Design review of the part built by this model. Coordinates are the model's own, in mm. Give positions to 0.01 mm unless a question says otherwise; leave off trailing zeros. Write each loop counter-clockwise with the first axis right and the second up, starting at its lowest first coordinate (ties: lowest second). Pieces come first, ordered by that corner, then holes. Notation, with made-up numbers: M -15,-13.5 L 5,-13.5 A14 ccw 5,-0.5 Z; hole C -9,-2 d6. An arc over 180 degrees is marked long. Answer in a Markdown table with one row per item.
```python
from build123d import *

# Parameters (mm, degrees)
BOARD_OUTLINE_DEPTH = 0.508
SKETCH2_R           = 0.0762
NPTH_DEPTH          = 1.508
SKETCH3_R           = 0.405
SKETCH3_R_2         = 1.27
PTH_DEPTH           = 1.508


with BuildPart() as part:
    # Sketch1 → Board_Outline (new body)
    with BuildSketch(Plane.XY):
        Polygon((0, 0), (0, 21.59), (0.3175, 23.1775), (14.2875, 23.1775), (14.605, 21.59), (14.605, 0), align=None)
    extrude(amount=BOARD_OUTLINE_DEPTH)

    # Sketch2 → NPTH (cut, through all)
    with BuildSketch(Plane.XY):
        with Locations((1.4224, 20.3073)):
            Circle(SKETCH2_R)
        with Locations((8.5344, 4.5593)):
            Circle(SKETCH2_R)
        with Locations((12.7, 17.5641)):
            Circle(SKETCH2_R)
        with Locations((12.065, 8.4582)):
            Circle(SKETCH2_R)
        with Locations((13.2842, 7.3406)):
            Circle(SKETCH2_R)
        with Locations((0.635, 14.732)):
            Circle(SKETCH2_R)
        with Locations((3.1496, 20.4089)):
            Circle(SKETCH2_R)
        with Locations((2.4384, 14.9225)):
            Circle(SKETCH2_R)
        with Locations((2.54, 20.4089)):
            Circle(SKETCH2_R)
        with Locations((2.54, 17.3609)):
            Circle(SKETCH2_R)
        with Locations((3.7592, 20.4089)):
            Circle(SKETCH2_R)
        with Locations((2.032, 14.4145)):
            Circle(SKETCH2_R)
        with Locations((4.3688, 20.4089)):
            Circle(SKETCH2_R)
        with Locations((2.4384, 13.9065)):
            Circle(SKETCH2_R)
        with Locations((5.08, 20.4089)):
            Circle(SKETCH2_R)
        with Locations((2.4384, 13.2969)):
            Circle(SKETCH2_R)
        with Locations((5.6896, 20.4089)):
            Circle(SKETCH2_R)
        with Locations((2.4384, 12.6873)):
            Circle(SKETCH2_R)
        with Locations((6.2992, 20.4089)):
            Circle(SKETCH2_R)
        with Locations((2.032, 12.1793)):
            Circle(SKETCH2_R)
        with Locations((6.9088, 20.4089)):
            Circle(SKETCH2_R)
        with Locations((2.4384, 11.6713)):
            Circle(SKETCH2_R)
        with Locations((7.62, 20.4089)):
            Circle(SKETCH2_R)
        with Locations((12.192, 11.6713)):
            Circle(SKETCH2_R)
        with Locations((12.0904, 20.4089)):
            Circle(SKETCH2_R)
        with Locations((12.0904, 17.4625)):
            Circle(SKETCH2_R)
        with Locations((11.4808, 20.4089)):
            Circle(SKETCH2_R)
        with Locations((12.192, 14.9225)):
            Circle(SKETCH2_R)
        with Locations((10.8712, 20.4089)):
            Circle(SKETCH2_R)
        with Locations((12.8016, 14.8209)):
            Circle(SKETCH2_R)
        with Locations((10.16, 20.4089)):
            Circle(SKETCH2_R)
        with Locations((12.5984, 14.0081)):
            Circle(SKETCH2_R)
        with Locations((9.5504, 20.4089)):
            Circle(SKETCH2_R)
        with Locations((12.192, 13.5001)):
            Circle(SKETCH2_R)
        with Locations((8.9408, 20.4089)):
            Circle(SKETCH2_R)
        with Locations((12.192, 12.8905)):
            Circle(SKETCH2_R)
        with Locations((8.3312, 20.4089)):
            Circle(SKETCH2_R)
        with Locations((12.192, 12.2809)):
            Circle(SKETCH2_R)
        with Locations((6.4008, 7.5057)):
            Circle(SKETCH2_R)
        with Locations((4.8768, 3.7465)):
            Circle(SKETCH2_R)
        with Locations((2.032, 5.0673)):
            Circle(SKETCH2_R)
        with Locations((5.2832, 6.5913)):
            Circle(SKETCH2_R)
        with Locations((7.62, 7.5057)):
            Circle(SKETCH2_R)
        with Locations((8.5344, 6.2865)):
            Circle(SKETCH2_R)
        with Locations((6.7056, 3.7465)):
            Circle(SKETCH2_R)
        with Locations((8.636, 7.5057)):
            Circle(SKETCH2_R)
        with Locations((9.2456, 7.5057)):
            Circle(SKETCH2_R)
        with Locations((8.128, 6.7945)):
            Circle(SKETCH2_R)
        with Locations((2.4384, 9.6393)):
            Circle(SKETCH2_R)
        with Locations((8.7376, 5.1689)):
            Circle(SKETCH2_R)
    extrude(amount=NPTH_DEPTH, mode=Mode.SUBTRACT)

    # Sketch3 → PTH (cut, through all)
    with BuildSketch(Plane.XY):
        with Locations((1.27, 8.57)):
            Circle(SKETCH3_R)
        with Locations((2.22, 1.59)):
            Circle(SKETCH3_R)
        with Locations((1.27, 10.48)):
            Circle(SKETCH3_R)
        with Locations((11.75, 2.86)):
            Circle(SKETCH3_R_2)
        with Locations((1.27, 6.67)):
            Circle(SKETCH3_R)
        with Locations((3.18, 6.67)):
            Circle(SKETCH3_R)
        with Locations((13.34, 16.51)):
            Circle(SKETCH3_R)
        with Locations((13.34, 11.43)):
            Circle(SKETCH3_R)
    extrude(amount=PTH_DEPTH, mode=Mode.SUBTRACT)


solid = part.part
```
1) Add section A-A (y = 16.51). Write out the cut boundary in (x, z) (3 decimals), and give its area (3 significant figures).
Geometry says:
| item | result |
|---|---|
| outline | M 0,0 L 12.935,0 L 12.935,0.508 L 0,0.508 Z; M 13.745,0 L 14.605,0 L 14.605,0.508 L 13.745,0.508 Z |
| area | 7.01 mm^2 |
2) The part is to be moulded in two halves that separate along X. For faces 1 (the face through (7, 12, 0)), 2 (the face through (0.95, 8.32, 0.25)), say which applies: released by +X, released by -X, zero draft, split by the parting line, or undercut.
Geometry says:
| item | result |
|---|---|
| face 1 | zero draft |
| face 2 | undercut |
3) Add section B-B (z = 0.3). Count the separate pieces of the cut face and the enclosed holes in it, and give its area (3 significant figures).
Geometry says:
| item | result |
|---|---|
| separate pieces | 1 |
| enclosed holes | 58 |
| area | 328 mm^2 |
4) To check wall thickness, follow probe 1 along Y at (x, z) = (8.75, 0.15); probe 2 along X at (y, z) = (3.25, 0.1) (3 decimals); probe 3 along X at (y, z) = (10.75, 0.2) (3 decimals). State the ranges of each line that lie inside material, in increasing order. Write a range as [from, to].
Geometry says:
| item | result |
|---|---|
| probe 1 | [0, 5.09], [5.24, 23.18] |
| probe 2 | [0, 10.541], [12.959, 14.605] |
| probe 3 | [0, 0.968], [1.572, 14.605] |
